The drawing under review shows one solid part. Ordinate dimensions are in mm from its lowest x, y, z. Round coordinates to 2 decimals unless told otherwise and drop trailing zeros. Write each loop counter-clockwise with the first axis right and the second up, starting at its lowest first coordinate (ties: lowest second). Pieces come first, ordered by that corner, then holes.
Item 1: Add section A-A (z = 28.5). Give the boundary of the cut face in (x, y).
Item 2: To check wall thickness, follow L1, parallel to Z at x = 40, y = 1.4 (1 decimal); L2, parallel to X at y = 2.2, z = 29.5 (1 decimal); L3, parallel to Z at x = 43, y = 0.85 (1 decimal). State the ranges of each line that lie inside material, in increasing order.
Item 3: Add section D-D (z = 37.5). Give the boundary of the cut face in (x, y).
Item 4: Clearance check with flat-ended pins moving along their axes: pin 1 Ø1.5 at (x, y) = (16.5, 0.5) entering from -Z (1 decimal); pin 2 Ø1.5 at (y, z) = (1.5, 26.5) entering from -X. State where each tip first meets the part, or that it passes through.
Item 5: Add section C-C (x = 26). Give the boundary of the cut face in (y, z) (1 decimal).
Item 6: Add section B-B (y = 1.7). Give the boundary of the cut face in (x, z) (1 decimal).
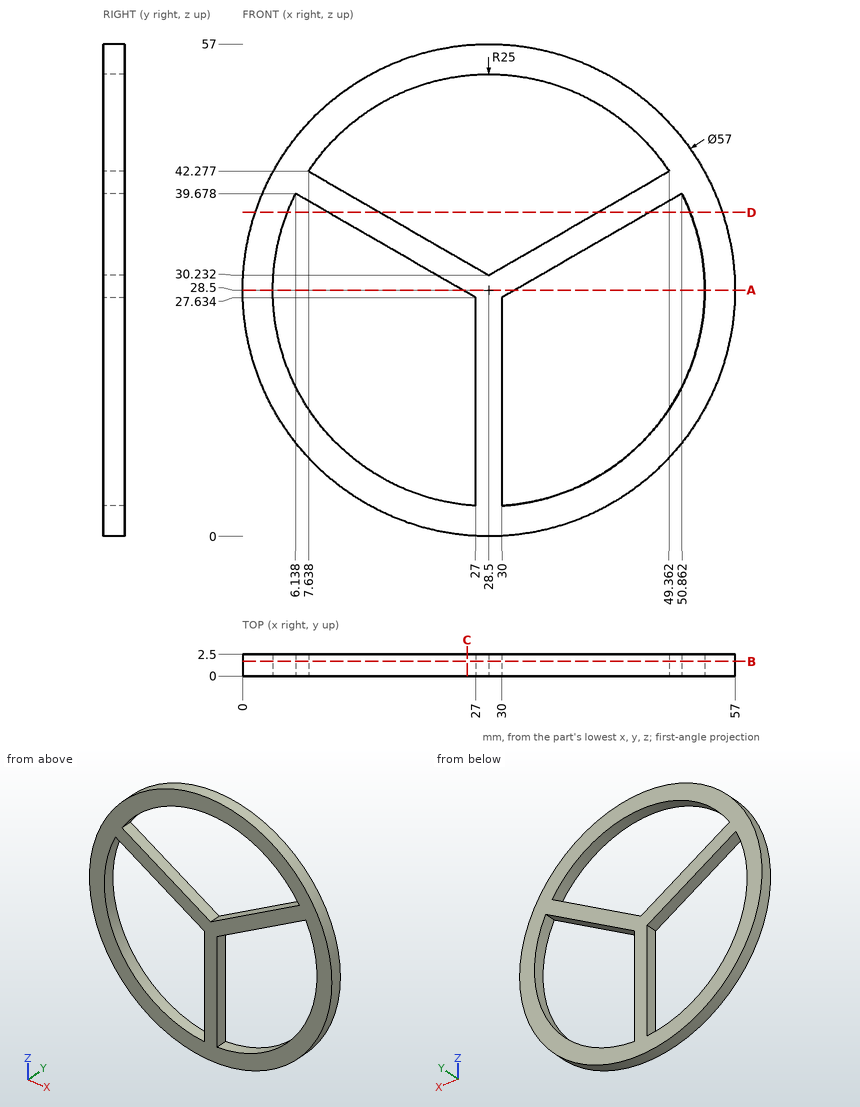
Numbers:
1. outline: (0, 0) - (3.5, 0) - (3.5, 2.5) - (0, 2.5) - close; (25.5, 0) - (31.5, 0) - (31.5, 2.5) - (25.5, 2.5) - close; (53.5, 0) - (57, 0) - (57, 2.5) - (53.5, 2.5) - close
2. L1: z = 2.4 to 6.3, 33.4 to 36.9, 50.7 to 54.6
2. L2: x = 0 to 3.5, 23.8 to 33.2, 53.5 to 57
2. L3: z = 4 to 8.1, 35.1 to 38.6, 48.9 to 53
3. outline: (1.46, 0) - (5.18, 0) - (5.18, 2.5) - (1.46, 2.5) - close; (9.91, 0) - (15.91, 0) - (15.91, 2.5) - (9.91, 2.5) - close; (41.09, 0) - (47.09, 0) - (47.09, 2.5) - (41.09, 2.5) - close; (51.82, 0) - (55.54, 0) - (55.54, 2.5) - (51.82, 2.5) - close
4. pin 1: stops at z = 2.3
4. pin 2: stops at x = 0.03
5. outline: (0, 0.1) - (2.5, 0.1) - (2.5, 3.6) - (0, 3.6) - close; (0, 28.2) - (2.5, 28.2) - (2.5, 31.7) - (0, 31.7) - close; (0, 53.4) - (2.5, 53.4) - (2.5, 56.9) - (0, 56.9) - close
6. outline: circle Ø57 at (28.5, 28.5); hole (6.1, 39.7) arc R25 ccw to (27, 3.5) - (27, 27.6) - close; hole (7.6, 42.3) - (28.5, 30.2) - (49.4, 42.3) arc R25 ccw to start; hole (30, 3.5) arc R25 ccw to (50.9, 39.7) - (30, 27.6) - close
